CAD build for the part. Positions are in the model's coordinates, mm. Face numbers are marked on the shaded views. A direction names the side the tool comes from. Round coordinates to 2 decimals unless told otherwise and drop trailing zeros. Order: outer loops, then holes, each group sorted by start corner. A loop starts at its lowest first (then second) coordinate and runs counter-clockwise, first axis right, second up. Notation, with made-up numbers: (-29.75, 47.25) - (-25.75, 47.25) arc R18 ccw to (-25.75, 78.25) - close; hole circle Ø7 at (-5.5, 68). An arc over 180 degrees is marked (long way). Write item = value, one per line.
from build123d import *

# Parameters (mm, degrees)
BASPROSKE_W         = 5
BASPROSKE_H         = 12.75
TOOTHCUT_DEPTH      = 19.711627401
TEETHCUTS_COUNT     = 15
TEETHCUTS_ANGLE     = 336
BORSKE_R            = 2.7
BORE_DEPTH          = 50.0015748
SKETCH1_R           = 2.7
BOSS_EXTRUDE1_DEPTH = 5
FILLET1_R           = 5


with BuildPart() as part:
    # BasProSke → Base-Revolve (revolve)
    with BuildSketch(Plane(origin=(0, 0, 0), x_dir=(1, 0, 0), z_dir=(0, 1, 0)), mode=Mode.PRIVATE) as base_revolve_sk:
        with Locations((2.5, 6.375)):
            Rectangle(BASPROSKE_W, BASPROSKE_H)
    revolve(base_revolve_sk.sketch.rotate(Axis((-10, 0, 0), (1, 0, 0)), 180), axis=Axis((-10, 0, 0), (1, 0, 0)))

    # TooCutSke → ToothCut (cut, through all)
    with BuildSketch(Plane(origin=(0, 0, 0), x_dir=(0, 0, -1), z_dir=(1, 0, 0))):
        with BuildLine():
            ThreePointArc((0.769645606, 9.34235097), (0, 9.374), (-0.769645606, 9.34235097))
            ThreePointArc((-0.769645606, 9.34235097), (-1.209019537, 11.113083179), (-2.315283452, 12.563849239))
            ThreePointArc((-2.315283452, 12.563849239), (0, 12.7754), (2.315283452, 12.563849239))
            ThreePointArc((2.315283452, 12.563849239), (1.209019537, 11.113083179), (0.769645606, 9.34235097))
        make_face()
    toothcut = extrude(amount=TOOTHCUT_DEPTH, mode=Mode.SUBTRACT)

    # TeethCuts: ToothCut ×15 about axis
    teethcuts_axis = Axis((-10, 0, 0), (1, 0, 0))
    for i in range(1, TEETHCUTS_COUNT):
        add(toothcut.rotate(teethcuts_axis, i * TEETHCUTS_ANGLE / (TEETHCUTS_COUNT - 1)), mode=Mode.SUBTRACT)

    # BorSke → Bore (cut, symmetric)
    with BuildSketch(Plane(origin=(0, 0, 0), x_dir=(0, 0, -1), z_dir=(1, 0, 0))):
        with Locations(Location((0, 0, 0), (0, 0, 180))):
            Circle(BORSKE_R)
    extrude(amount=BORE_DEPTH, both=True, mode=Mode.SUBTRACT)

    # Sketch1 → Boss-Extrude1 (add)
    with BuildSketch(Plane.ZY):
        with BuildLine():
            Line((4, 12.709543162), (4, 50))
            ThreePointArc((4, 50), (0, 54), (-4, 50))
            Line((-4, 50), (-4, 12.709543162))
            Line((-4, 12.709543162), (-7.194322072, 10.526358816))
            Line((-7.194322072, 10.526358816), (-4.502982719, 8.221619222))
            Line((-4.502982719, 8.221619222), (4.502982719, 8.221619222))
            Line((4.502982719, 8.221619222), (7.194322072, 10.526358816))
            Line((7.194322072, 10.526358816), (4, 12.709543162))
        make_face()
        with Locations((0, 50)):
            Circle(SKETCH1_R, mode=Mode.SUBTRACT)
    extrude(amount=-BOSS_EXTRUDE1_DEPTH)

    # Fillet1
    fillet1_edges = [part.edges().sort_by_distance(p)[0] for p in [
        (2.5, 12.709543162, 4),
        (2.5, 12.709543162, -4),
    ]]
    fillet(fillet1_edges, radius=FILLET1_R)


solid = part.part
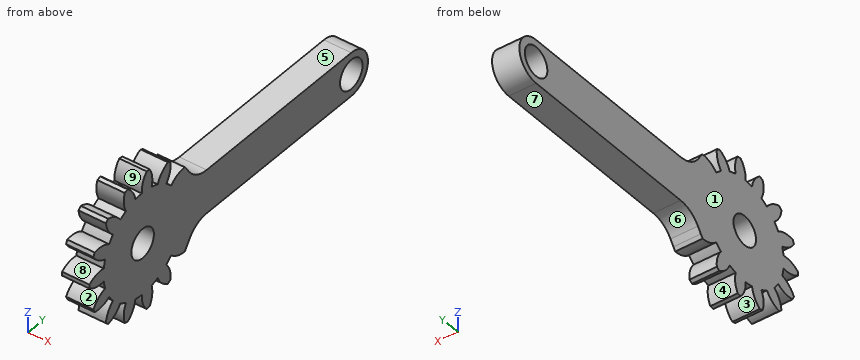
(1) Band-saw the part on C-C on y = 9. List the corners of the cut face in (x, z).
Solved:
outline = (0, -7.66) - (5, -7.66) - (5, 7.66) - (0, 7.66) - close
(2) Drop flat-ended pins along their axis: pin 1 (6 mm diameter, centred on y = 40, z = -1.5, fed in from -X); pin 2 (3 mm diameter, centred on x = 3.5, z = 6.5, fed in from -Y); pin 3 (1.5 mm diameter, centred on x = 1, z = -6.5, fed in from +Y). Give the stop position or say it passes through.
Solved:
pin_1 = 0
pin_2 = -11.73
pin_3 = 11.55
(3) Pull direction Y, two halves, no side cores. Call the marked faces 6, 7, 8 and 9: released by +Y, released by -Y, zero draft, split by the parting line, or undercut.
Solved:
face_6 = released by +Y
face_7 = zero draft
face_8 = undercut
face_9 = undercut
(4) Probe line 1 along Y through (x, z) = (2.1, 0); line 2 along Y through (x, z) = (1.3, 9.75); line 3 along Z through (x, y) = (1.8, 27.5). List the from-to ranges inside material, lowest first.
Solved:
line_1 = -12.75 to -2.7, 2.7 to 47.3, 52.7 to 54
line_2 = -4.45 to -1.85, -0.22 to 2.28, 4.21 to 6.68
line_3 = -4 to 4
(5) Tool access for the marked faces 1, 2, 3, 4 and 5: list every direction of +Z, -Z, +X, -X, +Y, -Y with a clear straight run to the whole face (end or side of a thin tool).
Solved:
face_1 = +Z, -Z, -X, +Y, -Y
face_2 = +X, -X, -Y
face_3 = -Z, +X, -X
face_4 = +X, -X
face_5 = +Z, +X, -X, +Y
(6) Band-saw the part on B-B on y = 24. List the corners of the cut face in (x, z).
Solved:
outline = (0, -4) - (5, -4) - (5, 4) - (0, 4) - close
(7) Band-saw the part on A-A on x = 1.7. Count the separate pieces of the cut face and the enclosed holes in it, plus the area to 3 significant figures.
Solved:
separate_pieces = 1
enclosed_holes = 2
area = 689 mm²
